```python
from build123d import *

# Parameters (mm, degrees)
SKETCH1_R               = 25
BOSS_EXTRUDE1_DEPTH     = 20
CUT_EXTRUDE1_DEPTH      = 41.620192023
CUT_EXTRUDE1_DEPTH_BACK = 41.620192023
SKETCH2_W               = 30
SKETCH2_H               = 10


with BuildPart() as part:
    # Sketch1 → Boss-Extrude1 (new body)
    with BuildSketch(Plane.XY):
        Circle(SKETCH1_R)
    extrude(amount=BOSS_EXTRUDE1_DEPTH)

    # Sketch2 → Cut-Extrude1 (cut, two sides: drawn at the far end of the back side and taken through both)
    with BuildSketch(Plane(origin=(0, 0, 0), x_dir=(0, 0, -1), z_dir=(1, 0, 0)).offset(-CUT_EXTRUDE1_DEPTH_BACK)):
        with Locations((-20, 0)):
            Rectangle(SKETCH2_W, SKETCH2_H)
    extrude(amount=CUT_EXTRUDE1_DEPTH + CUT_EXTRUDE1_DEPTH_BACK, mode=Mode.SUBTRACT)


solid = part.part
```
Geometry: final body of the model. Coordinates: model frame, mm. A direction names the side the tool comes from. Give positions to 0.01 mm unless a question says otherwise; leave off trailing zeros. Order: outer loops, then holes, each group sorted by start corner. A loop starts at its lowest first (then second) coordinate and runs counter-clockwise, first axis right, second up. Notation, with made-up numbers: M -7.5,3.5 L -2.5,3.5 A31 cw -2.5,38.5 Z; hole C 87,-16 d6. An arc over 180 degrees is marked long. Answer as CSV lines item,"result". Start each with the question number.
1) First-contact query: P1, Ø4, axis at y = 8.5, z = 14.5, coming from the -X side; P2, Ø8, axis at y = -12.5, z = 13.5, coming from the +X side; P3, Ø3, axis at x = -18, z = 4, coming from the +Y side. Flat tips, straight axial feed; report the tip coordinate or a pass-through.
2) Line query: line 1 (Y direction, x = -8, z = 12); line 2 (Y direction, x = -15, z = 12.5); line 3 (Y direction, x = 12.5, z = 4.25). Output: solid intervals per line, ascending. Write a range as from..to.
3) Set-up query: faces 1 (the flat face through (0, -5, 13)), 2 (the flat face through (0, 0, 0)). Return all of +Z, -Z, +X, -X, +Y, -Y with unobstructed straight access to the full face (end or side cutting, diameter ignored); none if empty.
4) Cut plane C-C (y = -15). Output: boundary loops of the cut face in (x, z).
5) Cut plane A-A (x = 0). Output: boundary loops of the cut face in (y, z), then the cut area to 3 significant figures.
6) Cut plane D-D (z = 2.75). Output: boundary loops of the cut face in (x, y).
7) Cut plane B-B (z = 12.5). Output: boundary loops of the cut face in (x, y).
8) Mould query, pull axis Y, two halves, no side actions, for faces 3 (the flat face through (0, 13, 20)), 4 (the cylindrical face through (23.846, 7.509, 9.86)), 5 (the flat face through (0, 5, 13)). Classes: +Y half, -Y half, draft (parallel to the pull), parting line (faces both ways), or undercut.
Findings below:
1,P1,"stops at x = -24.14"
1,P2,"stops at x = 23.51"
1,P3,"stops at y = 18.78"
2,line 1,"y = -23.69..-5, 5..23.69"
2,line 2,"y = -20..-5, 5..20"
2,line 3,"y = -21.65..21.65"
3,face 1,"+Z, +X, -X"
3,face 2,"-Z, +X, -X, +Y, -Y"
4,outline,"M -20,0 L 20,0 L 20,20 L -20,20 Z"
5,outline,"M -25,0 L 25,0 L 25,20 L 5,20 L 5,5 L -5,5 L -5,20 L -25,20 Z"
5,area,"850 mm²"
6,outline,"C 0,0 d50"
7,outline,"M -24.49,-5 A25 ccw 24.49,-5 Z; M -24.49,5 L 24.49,5 A25 ccw Z"
8,face 3,"draft"
8,face 4,"parting line"
8,face 5,"undercut"
